Source: CAD feature listing. Evaluate the final solid. Frame: model axes, mm. Coordinates: 2 decimals unless noted, no trailing zeros. Write each loop counter-clockwise with the first axis right and the second up, starting at its lowest first coordinate (ties: lowest second). Pieces come first, ordered by that corner, then holes. Notation, with made-up numbers: (10, -31) -> (27, -31) arc R15 cw to (27, -16) -> close; hole circle Ø11 at (-35.75, 73.5). An arc over 180 degrees is marked (long way). One line per item, written item: value. Start each with the question number.
1. Section query C-C, the plane z = -101.5. Output: boundary loops of the cut face in (x, y).
2. Section query B-B, the plane y = -2. Output: boundary loops of the cut face in (x, z).
3. First-contact query: P1, Ø6.5, axis at x = 0, z = -114.173, coming from the +Y side. Flat tip, straight axial feed; report the tip coordinate or a pass-through.
4. Section query A-A, the plane y = -19.5. Output: boundary loops of the cut face in (x, z), and give its area (3 significant figures).
5. Section query D-D, the plane z = 6.5. Output: boundary loops of the cut face in (x, y), and give its area (3 significant figures).
6. Line query: line 1 (Y direction, x = 8.5, z = -8); line 2 (X direction, y = -21, z = 0.5). Output: solid intervals per line, ascending.
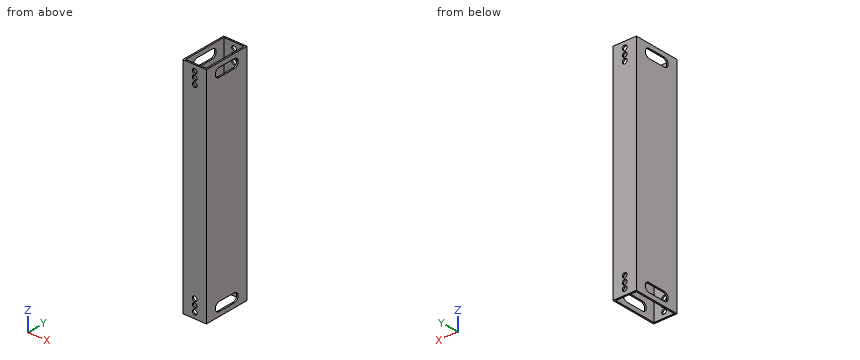
Autodesk Inventor part; units mm, degrees
ref_plane "YZ Plane" through (0, 0, 0) normal (1, 0, 0) x (0, 1, 0)
ref_plane "XZ Plane" through (0, 0, 0) normal (0, 1, 0) x (-1, 0, 0)
ref_plane "XY Plane" through (0, 0, 0) normal (0, 0, 1) x (1, 0, 0)
sketch "Sketch1" plane through (0, 0, 0) normal (0, 0, 1) x (1, 0, 0)
  line L0 (-12.7, -25.4) -> (12.7, -25.4)
  line L1 (12.7, -25.4) -> (12.7, 25.4)
  line L2 (12.7, 25.4) -> (-12.7, 25.4)
  line L3 (-12.7, 25.4) -> (-12.7, -25.4)
  line L4 (-12.7, -25.4) -> (12.7, 25.4) construction
  line L5 (12.7, -25.4) -> (-12.7, 25.4) construction
  line L6 (-11.1125, 23.8125) -> (11.1125, 23.8125)
  line L7 (11.1125, 23.8125) -> (11.1125, -23.8125)
  line L8 (11.1125, -23.8125) -> (-11.1125, -23.8125)
  line L9 (-11.1125, -23.8125) -> (-11.1125, 23.8125)
  point P0 (0, 0)
  dimension "width" = 25.4
  dimension "height" = 50.8
  dimension "thickness" = 1.5875
extrude "Extrusion1" add sketch "Sketch1" along normal mid plane 241.046
sketch "Sketch3" plane through (-12.7, 25.4, 120.523) normal (0, 1, 0) x (1, 0, 0)
  line L0 (25.4, 0) -> (0, 0)
  line L1 (0, 241.046) -> (0, 0) construction
  line L2 (0, 241.046) -> (25.4, 241.046) construction
  point P0 (12.7, 120.523)
  point P1 (12.7, 6.35)
  point P2 (12.7, 12.7)
  point P3 (12.7, 19.05)
  point P4 (12.7, 234.696)
  point P5 (12.7, 228.346)
  point P6 (12.7, 221.996)
  dimension "d18" = 6.35
  dimension "d19" = 6.35
  dimension "d20" = 6.35
  dimension "d21" = 12.7
  dimension "d22" = 6.35
  dimension "d23" = 6.35
  dimension "d24" = 6.35
hole "Hole2" at (0, 25.4, 114.173) at (0, 25.4, 107.823) at (0, 25.4, 101.473) at (0, 25.4, -101.473) at (0, 25.4, -107.823) at (0, 25.4, -114.173) direction (0, -1, 0) diameter 5.1054 end through all
sketch "Sketch4" plane through (12.7, -25.4, 120.523) normal (1, 0, 0) x (0, 0, -1)
  line L0 (9.525, 34.925) -> (9.525, 15.875) construction
  line L1 (4.7625, 34.925) -> (4.7625, 15.875)
  line L2 (14.2875, 15.875) -> (14.2875, 34.925)
  arc A0 (14.2875, 34.925) -> (4.7625, 34.925) centre (9.525, 34.925) ccw
  arc A1 (4.7625, 15.875) -> (14.2875, 15.875) centre (9.525, 15.875) ccw
  line L3 (0, 0) -> (0, 50.8) construction
  line L4 (120.523, 25.4) -> (120.523, 50.8) construction
  line L5 (241.046, 50.8) -> (0, 50.8) construction
  line L6 (231.521, 34.925) -> (231.521, 15.875) construction
  line L7 (236.2835, 34.925) -> (236.2835, 15.875)
  line L8 (226.7585, 15.875) -> (226.7585, 34.925)
  arc A2 (236.2835, 34.925) -> (226.7585, 34.925) centre (231.521, 34.925) ccw
  arc A3 (226.7585, 15.875) -> (236.2835, 15.875) centre (231.521, 15.875) ccw
  point P0 (9.525, 25.4)
  point P1 (231.521, 25.4)
  dimension "d32" = 9.525
  dimension "d33" = 19.05
  dimension "d34" = 9.525
extrude "Extrusion2" cut sketch "Sketch4" against normal through all
properties part number "EL2-011" material "Aluminum 6061"
Computed values:
1. outline: (-12.7, -25.4) -> (-2.55, -25.4) -> (-2.55, -23.81) -> (-11.11, -23.81) -> (-11.11, 23.81) -> (-2.55, 23.81) -> (-2.55, 25.4) -> (-12.7, 25.4) -> close; (2.55, -25.4) -> (12.7, -25.4) -> (12.7, 25.4) -> (2.55, 25.4) -> (2.55, 23.81) -> (11.11, 23.81) -> (11.11, -23.81) -> (2.55, -23.81) -> close
2. outline: (-12.7, -120.52) -> (-11.11, -120.52) -> (-11.11, -115.76) -> (-12.7, -115.76) -> close; (-12.7, -106.24) -> (-11.11, -106.24) -> (-11.11, 106.24) -> (-12.7, 106.24) -> close; (-12.7, 115.76) -> (-11.11, 115.76) -> (-11.11, 120.52) -> (-12.7, 120.52) -> close; (11.11, -120.52) -> (12.7, -120.52) -> (12.7, -115.76) -> (11.11, -115.76) -> close; (11.11, -106.24) -> (12.7, -106.24) -> (12.7, 106.24) -> (11.11, 106.24) -> close; (11.11, 115.76) -> (12.7, 115.76) -> (12.7, 120.52) -> (11.11, 120.52) -> close
3. P1: stops at y = 25.4
4. outline: (-12.7, -120.52) -> (-11.11, -120.52) -> (-11.11, 120.52) -> (-12.7, 120.52) -> close; (11.11, -120.52) -> (12.7, -120.52) -> (12.7, 120.52) -> (11.11, 120.52) -> close
4. area: 765 mm²
5. outline: (-12.7, -25.4) -> (12.7, -25.4) -> (12.7, 25.4) -> (-12.7, 25.4) -> close; hole (-11.11, -23.81) -> (11.11, -23.81) -> (11.11, 23.81) -> (-11.11, 23.81) -> close
5. area: 232 mm²
6. line 1: y = -25.4 to -23.81, 23.81 to 25.4
6. line 2: x = -12.7 to -11.11, 11.11 to 12.7
